```python
from build123d import *

# Parameters (mm, degrees)
SKETCH1_W           = 400
SKETCH1_H           = 250
SKETCH1_W_2         = 15
SKETCH1_H_2         = 3.2
SKETCH1_W_3         = 3.2
SKETCH1_H_3         = 15
BOSS_EXTRUDE2_DEPTH = 3
FILLET1_R           = 10
SKETCH2_R           = 2
SKETCH2_R_2         = 1
SKETCH2_R_3         = 4
CUT_EXTRUDE1_DEPTH  = 472.708596487


with BuildPart() as part:
    # Sketch1 → Boss-Extrude2 (new body)
    with BuildSketch(Plane(origin=(0, 0, 0), x_dir=(1, 0, 0), z_dir=(0, 1, 0))):
        with Locations((200, 125)):
            Rectangle(SKETCH1_W, SKETCH1_H)
        with Locations((90, 4.6)):
            Rectangle(SKETCH1_W_2, SKETCH1_H_2, mode=Mode.SUBTRACT)
        with Locations((35, 4.6)):
            Rectangle(SKETCH1_W_2, SKETCH1_H_2, mode=Mode.SUBTRACT)
        with Locations((145, 4.6)):
            Rectangle(SKETCH1_W_2, SKETCH1_H_2, mode=Mode.SUBTRACT)
        with Locations((200, 4.6)):
            Rectangle(SKETCH1_W_2, SKETCH1_H_2, mode=Mode.SUBTRACT)
        with Locations((255, 4.6)):
            Rectangle(SKETCH1_W_2, SKETCH1_H_2, mode=Mode.SUBTRACT)
        with Locations((310, 4.6)):
            Rectangle(SKETCH1_W_2, SKETCH1_H_2, mode=Mode.SUBTRACT)
        with Locations((365, 4.6)):
            Rectangle(SKETCH1_W_2, SKETCH1_H_2, mode=Mode.SUBTRACT)
        with Locations((365, 245.4)):
            Rectangle(SKETCH1_W_2, SKETCH1_H_2, mode=Mode.SUBTRACT)
        with Locations((310, 245.4)):
            Rectangle(SKETCH1_W_2, SKETCH1_H_2, mode=Mode.SUBTRACT)
        with Locations((255, 245.4)):
            Rectangle(SKETCH1_W_2, SKETCH1_H_2, mode=Mode.SUBTRACT)
        with Locations((200, 245.4)):
            Rectangle(SKETCH1_W_2, SKETCH1_H_2, mode=Mode.SUBTRACT)
        with Locations((35, 245.4)):
            Rectangle(SKETCH1_W_2, SKETCH1_H_2, mode=Mode.SUBTRACT)
        with Locations((90, 245.4)):
            Rectangle(SKETCH1_W_2, SKETCH1_H_2, mode=Mode.SUBTRACT)
        with Locations((145, 245.4)):
            Rectangle(SKETCH1_W_2, SKETCH1_H_2, mode=Mode.SUBTRACT)
        with Locations((11.6, 95)):
            Rectangle(SKETCH1_W_3, SKETCH1_H_3, mode=Mode.SUBTRACT)
        with Locations((11.6, 35)):
            Rectangle(SKETCH1_W_3, SKETCH1_H_3, mode=Mode.SUBTRACT)
        with Locations((11.6, 155)):
            Rectangle(SKETCH1_W_3, SKETCH1_H_3, mode=Mode.SUBTRACT)
        with Locations((11.6, 215)):
            Rectangle(SKETCH1_W_3, SKETCH1_H_3, mode=Mode.SUBTRACT)
        with Locations((388.4, 35)):
            Rectangle(SKETCH1_W_3, SKETCH1_H_3, mode=Mode.SUBTRACT)
        with Locations((388.4, 95)):
            Rectangle(SKETCH1_W_3, SKETCH1_H_3, mode=Mode.SUBTRACT)
        with Locations((388.4, 155)):
            Rectangle(SKETCH1_W_3, SKETCH1_H_3, mode=Mode.SUBTRACT)
        with Locations((388.4, 215)):
            Rectangle(SKETCH1_W_3, SKETCH1_H_3, mode=Mode.SUBTRACT)
    extrude(amount=BOSS_EXTRUDE2_DEPTH)

    # Fillet1
    fillet1_edges = [part.edges().sort_by_distance(p)[0] for p in [
        (0, 1.5, -250),
        (400, 1.5, -250),
        (400, 1.5, 0),
        (0, 1.5, 0),
    ]]
    fillet(fillet1_edges, radius=FILLET1_R)

    # Sketch2 → Cut-Extrude1 (cut, through all)
    with BuildSketch(Plane(origin=(0, 3, 0), x_dir=(1, 0, 0), z_dir=(0, 1, 0))):
        with Locations(Location((89.493903346, 135.606601718, 0), (0, 0, 270))):
            Circle(SKETCH2_R)
        with Locations(Location((120.606601718, 145.506096654, 0), (0, 0, 270))):
            Circle(SKETCH2_R)
        with Locations(Location((130.506096654, 135.606601718, 0), (0, 0, 270))):
            Circle(SKETCH2_R)
        with Locations(Location((99.393398282, 104.493903346, 0), (0, 0, 270))):
            Circle(SKETCH2_R)
        with Locations(Location((120.606601718, 104.493903346, 0), (0, 0, 270))):
            Circle(SKETCH2_R)
        with Locations(Location((89.493903346, 114.393398282, 0), (0, 0, 270))):
            Circle(SKETCH2_R)
        with Locations(Location((81, 119.62, 0), (0, 0, 270))):
            Circle(SKETCH2_R_2)
        with Locations(Location((110, 125, 0), (0, 0, 270))):
            Circle(SKETCH2_R_3)
        with Locations(Location((81, 130.38, 0), (0, 0, 270))):
            Circle(SKETCH2_R_2)
        with Locations(Location((99.393398282, 145.506096654, 0), (0, 0, 270))):
            Circle(SKETCH2_R)
        with Locations(Location((104.62, 154, 0), (0, 0, 270))):
            Circle(SKETCH2_R_2)
        with Locations(Location((115.38, 154, 0), (0, 0, 270))):
            Circle(SKETCH2_R_2)
        with Locations(Location((139, 130.38, 0), (0, 0, 270))):
            Circle(SKETCH2_R_2)
        with Locations(Location((139, 119.62, 0), (0, 0, 270))):
            Circle(SKETCH2_R_2)
        with Locations(Location((130.506096654, 114.393398282, 0), (0, 0, 270))):
            Circle(SKETCH2_R)
        with Locations(Location((115.38, 96, 0), (0, 0, 270))):
            Circle(SKETCH2_R_2)
        with Locations(Location((104.62, 96, 0), (0, 0, 270))):
            Circle(SKETCH2_R_2)
    extrude(amount=-CUT_EXTRUDE1_DEPTH, mode=Mode.SUBTRACT)


solid = part.part
```
Here's how the part is built. I have some questions about the finished solid (model axes, mm). Give positions to 0.01 mm unless a question says otherwise; leave off trailing zeros. Order: outer loops, then holes, each group sorted by start corner. A loop starts at its lowest first (then second) coordinate and runs counter-clockwise, first axis right, second up. Notation, with made-up numbers: (71.25, -32.5) -> (81.25, -32.5) arc R28 cw to (81.25, -5.5) -> close; hole circle Ø5 at (-23, 18). An arc over 180 degrees is marked (long way). Use CSV: the item, a comma, the result in double quotes. Start each with the question number.
Item 1: I'm going to push flat-ended pins straight in: P1, Ø3, axis at x = 115.38, z = -96, coming from the -Y side; P2, Ø1.5, axis at y = 1.5, z = -4, coming from the +X side. Where does each tip first touch, or does it pass through?
Item 2: Suppose I cut it at C-C (z = -125). List the corners of the cut face in (x, y) for me, and give its area (3 significant figures).
Item 3: Suppose I cut it at B-B (x = 110). List the corners of the cut face in (y, z) for me, and give its area (3 significant figures).
Item 4: Suppose I cut it at A-A (z = -216). List the corners of the cut face in (x, y) for me, and give its area (3 significant figures).
Item 5: If I drill on probe 1 along Z at (x, y) = (194, 2.2); probe 2 along X at (y, z) = (1, -135.5); probe 3 along X at (y, z) = (2, -96), over which ranges is the centre line in solid material (lowest first)? Write a range as [from, to].
Item 6: Thinking about a two-plate mould opening in Z: for faces 1 (the cylindrical face through (396.99, 1.52, -247.15)), 2 (the cylindrical face through (113.966, 1.521, -125.521)), 3 (the cylindrical face through (396.99, 1.52, -2.85)), which applies, pulls with the +Z half, pulls with the -Z half, needs draft (parallel to the pull), parting line crosses it, or undercut?
Answer block:
1,P1,"stops at y = 0"
1,P2,"stops at x = 398.51"
2,outline,"(0, 0) -> (106, 0) -> (106, 3) -> (0, 3) -> close; (114, 0) -> (400, 0) -> (400, 3) -> (114, 3) -> close"
2,area,"1,180 mm^2"
3,outline,"(0, -250) -> (3, -250) -> (3, -129) -> (0, -129) -> close; (0, -121) -> (3, -121) -> (3, 0) -> (0, 0) -> close"
3,area,"726 mm^2"
4,outline,"(0, 0) -> (10, 0) -> (10, 3) -> (0, 3) -> close; (13.2, 0) -> (386.8, 0) -> (386.8, 3) -> (13.2, 3) -> close; (390, 0) -> (400, 0) -> (400, 3) -> (390, 3) -> close"
4,area,"1,180 mm^2"
5,probe 1,"z = [-250, -247], [-243.8, -6.2], [-3, 0]"
5,probe 2,"x = [0, 87.5], [91.49, 128.51], [132.5, 400]"
5,probe 3,"x = [0, 10], [13.2, 103.62], [105.62, 114.38], [116.38, 386.8], [390, 400]"
6,face 1,"pulls with the -Z half"
6,face 2,"undercut"
6,face 3,"pulls with the +Z half"
